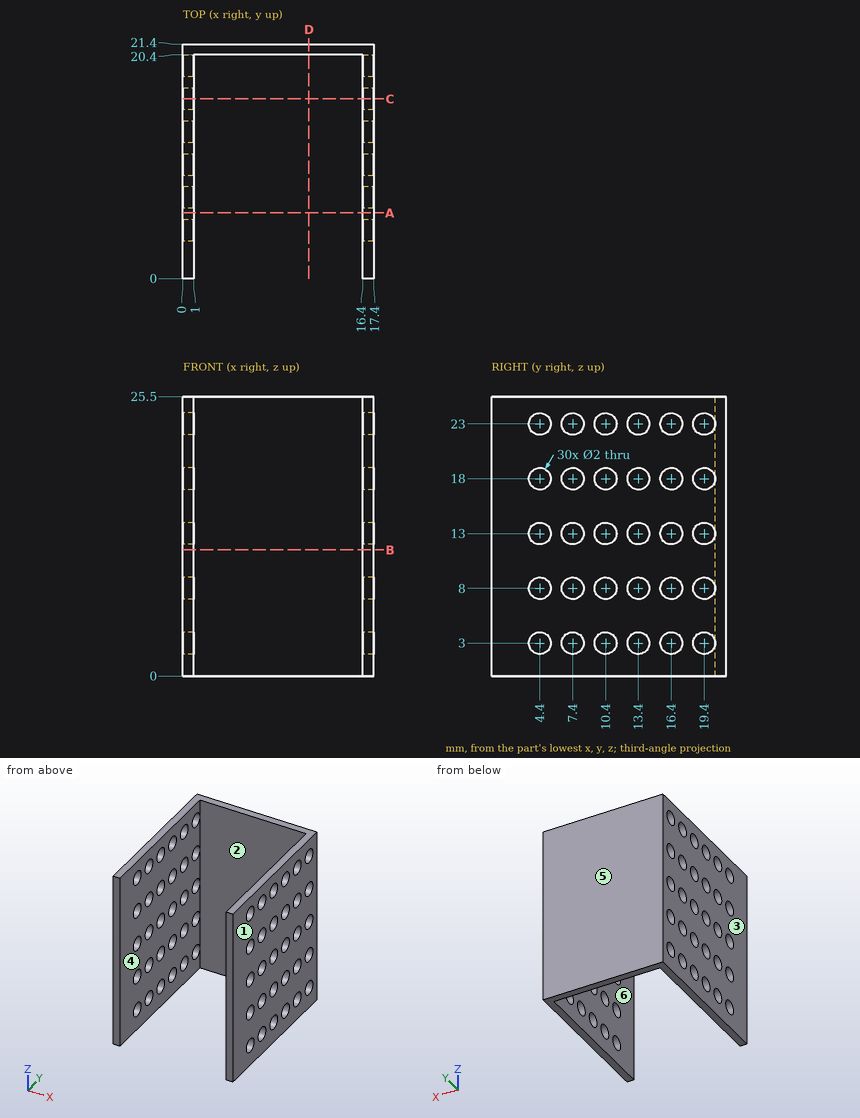
Input: dimensioned drawing with shaded views. Units: mm. Origin: part minimum x, y, z. A direction names the side the tool comes from. Coordinates: 2 decimals unless noted, no trailing zeros. Loops run counter-clockwise (first coordinate to the right, second up) from the corner with the lowest first, then second, coordinate; pieces in that order, holes last. Notation, with made-up numbers: (85.25, 85.25) -> (92.25, 85.25) arc R18 ccw to (92.25, 91.25) -> close; hole circle Ø1 at (-1, 47.25). An arc over 180 degrees is marked (long way). Use a Markdown table: item, result. Add a question column.
(1) Section query C-C, the plane y = 16.4. State how many separate pieces and enclosed holes the cut face has, plus the area to 3 significant figures.
(2) Access query for the marked faces 1 and 2. Directions: +Z, -Z, +X, -X, +Y, -Y. A direction counts if a zero-diameter tool reaches every point of the face in a straight line with its end or side. Return the directions, or none.
(3) Section query A-A, the plane y = 6. Return loops of the section in (x, z), plus the area to 3 significant figures.
(4) Mould query, pull axis X, two halves, no side actions, for the marked faces 3, 4, 5 and 6. Classes: pulls with the +X half, pulls with the -X half, needs draft (parallel to the pull), parting line crosses it, or undercut.
(5) Section query D-D, the plane x = 11.5. Return loops of the section in (y, z).
(6) Line query: line 1 along Z through (x, y) = (17.25, 16.4); line 2 along X through (y, z) = (16.75, 1.5); line 3 along Y through (x, z) = (16, 1.75). Output: solid intervals per line, ascending.
(7) Section query B-B, the plane z = 11.5. Return loops of the section in (x, y).
Answer:
| question | item | result |
|---|---|---|
| 1 | separate pieces | 12 |
| 1 | enclosed holes | 0 |
| 1 | area | 31.0 mm^2 |
| 2 | face 1 | +Z, -Z, +X, +Y, -Y |
| 2 | face 2 | +Z, -Z, -Y |
| 3 | outline | (0, 0) -> (1, 0) -> (1, 25.5) -> (0, 25.5) -> close; (16.4, 0) -> (17.4, 0) -> (17.4, 25.5) -> (16.4, 25.5) -> close |
| 3 | area | 51.0 mm^2 |
| 4 | face 3 | pulls with the -X half |
| 4 | face 4 | undercut |
| 4 | face 5 | needs draft |
| 4 | face 6 | undercut |
| 5 | outline | (20.4, 0) -> (21.4, 0) -> (21.4, 25.5) -> (20.4, 25.5) -> close |
| 6 | line 1 | z = 0 to 2, 4 to 7, 9 to 12, 14 to 17, 19 to 22, 24 to 25.5 |
| 6 | line 2 | x = 0 to 1, 16.4 to 17.4 |
| 6 | line 3 | y = 20.4 to 21.4 |
| 7 | outline | (0, 0) -> (1, 0) -> (1, 20.4) -> (16.4, 20.4) -> (16.4, 0) -> (17.4, 0) -> (17.4, 21.4) -> (0, 21.4) -> close |
